Read the model definition and answer for the solid it produces. Units are mm, in the model's axes. A direction names the side the tool comes from. Give positions to 0.01 mm unless a question says otherwise; leave off trailing zeros. Loops run counter-clockwise (first coordinate to the right, second up) from the corner with the lowest first, then second, coordinate; pieces in that order, holes last. Notation, with made-up numbers: (61.25, -21.5) -> (113.25, -21.5) arc R20 cw to (113.25, 4.5) -> close; hole circle Ø2 at (7.5, 17). An arc over 180 degrees is marked (long way). Return JSON: item names as keys, results as strings. Group by question number.
from build123d import *

# Parameters (mm, degrees)
SKETCH_1_W          = 23.8
SKETCH_1_H          = 7.8
EXTRUDE_1_DEPTH     = 3.2
SKETCH_2_R          = 2.4
EXTRUDE_2_DEPTH     = 1.7
SKETCH_3_R          = 2.5
CUT_EXTRUDE_1_DEPTH = 1.8


with BuildPart() as part:
    # Эскиз1 → Бобышка-Вытянуть1 (new body)
    with BuildSketch(Plane.XY):
        Rectangle(SKETCH_1_W, SKETCH_1_H)
    extrude(amount=EXTRUDE_1_DEPTH)

    # Эскиз2 → Бобышка-Вытянуть2 (add)
    with BuildSketch(Plane(origin=(0, 0, 0), x_dir=(-1, 0, 0), z_dir=(0, 0, -1))):
        Circle(SKETCH_2_R)
        with Locations((8, 0)):
            Circle(SKETCH_2_R)
        with Locations((-8, 0)):
            Circle(SKETCH_2_R)
    extrude(amount=EXTRUDE_2_DEPTH)

    # Эскиз3 → Вырез-Вытянуть1 (cut)
    with BuildSketch(Plane.XY.offset(3.2)):
        Circle(SKETCH_3_R)
        with Locations((-8, -0.211129939)):
            Circle(SKETCH_3_R)
        with Locations((8, 0)):
            Circle(SKETCH_3_R)
    extrude(amount=-CUT_EXTRUDE_1_DEPTH, mode=Mode.SUBTRACT)


solid = part.part
1. Determine the mould class of faces 1 (the flat face through (0, -3.9, 2)), 2 (the flat face through (-11.9, 0, 2)), 3 (the cylindrical face through (10.398, 0.106, -0.838)), 4 (the flat face through (11.9, 0, 2)) for opening direction X: pulls with the +X half, pulls with the -X half, needs draft (parallel to the pull), parting line crosses it, or undercut.
2. Which of the six approach directions +Z, -Z, +X, -X, +Y, -Y give full straight-line access (tool end or side, diameter ignored) to faces 5 (the flat face through (8, 0, 1.4)), 6 (the cylindrical face through (-9.29, 2.024, -0.838)), 7 (the flat face through (0, 3, 3.2))?
3. Section C-C on y = 3.25 is taken. Determine the outline of the cut face in (x, z), then the cut area to 3 significant figures.
4. Section B-B on y = 1.5 is taken. Determine the outline of the cut face in (x, z), then the cut area to 3 significant figures.
5. Section D-D on x = -4 is taken. Determine the outline of the cut face in (y, z), then the cut area to 3 significant figures.
6. Straight lines are drawn through the part: line 1 (Y direction, x = 0, z = 2.6); line 2 (Y direction, x = -8, z = 2.4); line 3 (Z direction, x = -1, y = -2.5). For each, find the intervals that lie inside material, in ascending order. Write a range as from..to.
7. A flat-ended cylindrical pin translates along its axis: pin 1 Ø4.5 at (x, y) = (8, 0) entering from +Z. Find the tip coordinate at first contact, or state that the pin passes through.
8. Section A-A on x = 8 is taken. Determine the outline of the cut face in (y, z), then the cut area to 3 significant figures.
Completed:
{
 "1": {"face 1": "needs draft", "face 2": "pulls with the -X half", "face 3": "undercut", "face 4": "pulls with the +X half"},
 "2": {"face 5": "+Z", "face 6": "-Z", "face 7": "+Z, +X, -X, +Y, -Y"},
 "3": {"outline": "(-11.9, 0) -> (11.9, 0) -> (11.9, 3.2) -> (-11.9, 3.2) -> close", "area": "76.2 mm²"},
 "4": {"outline": "(-11.9, 0) -> (-9.87, 0) -> (-9.87, -1.7) -> (-6.13, -1.7) -> (-6.13, 0) -> (-1.87, 0) -> (-1.87, -1.7) -> (1.87, -1.7) -> (1.87, 0) -> (6.13, 0) -> (6.13, -1.7) -> (9.87, -1.7) -> (9.87, 0) -> (11.9, 0) -> (11.9, 3.2) -> (10, 3.2) -> (10, 1.4) -> (6, 1.4) -> (6, 3.2) -> (2, 3.2) -> (2, 1.4) -> (-2, 1.4) -> (-2, 3.2) -> (-6.18, 3.2) -> (-6.18, 1.4) -> (-9.82, 1.4) -> (-9.82, 3.2) -> (-11.9, 3.2) -> close", "area": "74.3 mm²"},
 "5": {"outline": "(-3.9, 0) -> (3.9, 0) -> (3.9, 3.2) -> (-3.9, 3.2) -> close", "area": "25.0 mm²"},
 "6": {"line 1": "y = -3.9..-2.5, 2.5..3.9", "line 2": "y = -3.9..-2.71, 2.29..3.9", "line 3": "z = 0..3.2"},
 "7": {"pin 1": "stops at z = 1.4"},
 "8": {"outline": "(-3.9, 0) -> (-2.4, 0) -> (-2.4, -1.7) -> (2.4, -1.7) -> (2.4, 0) -> (3.9, 0) -> (3.9, 3.2) -> (2.5, 3.2) -> (2.5, 1.4) -> (-2.5, 1.4) -> (-2.5, 3.2) -> (-3.9, 3.2) -> close", "area": "24.1 mm²"}
}
